Check sheet for the modelled part. Datum: model origin and axes. Units: mm. A direction names the side the tool comes from. Give positions to 0.01 mm unless a question says otherwise; leave off trailing zeros. Use CSV: the item, a comma, the result in double quotes. Start each with the question number.
1. Access from +Z, -Z, +X, -X, +Y, -Y to the whole of each face (thin tool, end or side, straight path). Record for faces 3 (the face through (35, 6, -5)), 4 (the face through (44.84, 9.89, -2.46)), 5 (the face through (30, 2, -2)).
2. Scan lines: line 1 (X direction, y = 2.75, z = -0.75); line 2 (Y direction, x = 37.5, z = -2.7); line 3 (Y direction, x = 47, z = -4.5). Record each from-to range of solid material in increasing order.
3. Mould release check, pull along X, two halves, no side actions. Record for faces 1 (the face through (35, 6, 0)), 2 (the face through (66.833, 9.891, -2.465)): +X half, -X half, draft (parallel to the pull), parting line (faces both ways), or undercut.
4. Depth check by flat-ended pin: P1, Ø1.5, axis at x = 37, z = -3, coming from the -Y side. Enter the tip coordinate at first touch or a pass-through.
from build123d import *

# Parameters (mm, degrees)
BLANKSKE_W          = 70
BLANKSKE_H          = 11
BLANK_DEPTH         = 5
TOOTHCUTSIM_DEPTH   = 72.035202541
TEETHCUTS_COUNT     = 23
TEETHCUTS_PITCH     = 3.14159265
SKETCH_1_W          = 10
SKETCH_1_H          = 5
CUT_EXTRUDE_1_DEPTH = 72.035202541


with BuildPart() as part:
    # BlankSke → Blank (new body)
    with BuildSketch(Plane.XY):
        with Locations((35, 5.5)):
            Rectangle(BLANKSKE_W, BLANKSKE_H)
    extrude(amount=-BLANK_DEPTH)

    # TooCutSkeSim → ToothCutSim (cut, through all)
    with BuildSketch(Plane.XY):
        Polygon((0.44443537, 8.75), (-0.44443537, 8.75), (-1.272613241, 11.0254), (1.272613241, 11.0254), align=None)
    toothcutsim = extrude(amount=-TOOTHCUTSIM_DEPTH, mode=Mode.SUBTRACT)

    # TeethCuts: ToothCutSim ×23
    with Locations(*[(i * TEETHCUTS_PITCH, 0, 0) for i in range(1, TEETHCUTS_COUNT)]):
        add(toothcutsim, mode=Mode.SUBTRACT)

    # ｽｹｯﾁ1 → ｶｯﾄ - 押し出し1 (cut, through all)
    with BuildSketch(Plane.XY):
        with Locations((15, 2.5)):
            Rectangle(SKETCH_1_W, SKETCH_1_H)
        with Locations((35, 2.5)):
            Rectangle(SKETCH_1_W, SKETCH_1_H)
        with Locations((55, 2.5)):
            Rectangle(SKETCH_1_W, SKETCH_1_H)
    extrude(amount=-CUT_EXTRUDE_1_DEPTH, mode=Mode.SUBTRACT)


solid = part.part
Worked answers:
1,face 3,"-Z, +X, -X, +Y, -Y"
1,face 4,"+Z, -Z, +Y"
1,face 5,"+Z, -Z, -Y"
2,line 1,"x = 0 to 10, 20 to 30, 40 to 50, 60 to 70"
2,line 2,"y = 5 to 8.75"
2,line 3,"y = 0 to 8.75"
3,face 1,"draft"
3,face 2,"undercut"
4,P1,"stops at y = 5"
